Source: CAD feature listing. Evaluate the final solid. Frame: model axes, mm. A direction names the side the tool comes from. Coordinates: 2 decimals unless noted, no trailing zeros. Order: outer loops, then holes, each group sorted by start corner. A loop starts at its lowest first (then second) coordinate and runs counter-clockwise, first axis right, second up.
```python
from build123d import *

# Parameters (mm, degrees)
SKETCH2_R           = 14.5
BOSS_EXTRUDE1_DEPTH = 220
FILLET1_R           = 5
SKETCH3_R           = 19.5
BOSS_EXTRUDE2_DEPTH = 5
FILLET2_R           = 1


with BuildPart() as part:
    # Sketch2 → Boss-Extrude1 (new body)
    with BuildSketch(Plane(origin=(0, 0, 0), x_dir=(1, 0, 0), z_dir=(0, 1, 0))):
        with Locations(Location((0, 0, 0), (0, 0, 270))):
            Circle(SKETCH2_R)
    extrude(amount=BOSS_EXTRUDE1_DEPTH)

    # Fillet1
    fillet1_edges = [part.edges().sort_by_distance(p)[0] for p in [
        (0, 220, -14.5),
    ]]
    fillet(fillet1_edges, radius=FILLET1_R)

    # Sketch3 → Boss-Extrude2 (add)
    with BuildSketch(Plane.XZ):
        with Locations(Location((0, 0, 0), (0, 0, 270))):
            Circle(SKETCH3_R)
    extrude(amount=-BOSS_EXTRUDE2_DEPTH)

    # Fillet2
    fillet2_edges = [part.edges().sort_by_distance(p)[0] for p in [
        (0, 5, 19.5),
        (0, 0, 19.5),
        (0, 5, -14.5),
    ]]
    fillet(fillet2_edges, radius=FILLET2_R)


solid = part.part
```
Q1. Material intervals for line 1 along Y through (x, z) = (-11.5, -13); line 2 along X through (y, z) = (149, -1); line 3 along Y through (x, z) = (11, 8), sorted ascending.
Solutions:
line 1: y = 0 to 5
line 2: x = -14.47 to 14.47
line 3: y = 0 to 217.86
Q2. Section query A-A on x = 0. Output: boundary loops of the cut face in (y, z).
Solutions:
outline: (0, -18.5) arc R1 ccw to (1, -19.5) - (4, -19.5) arc R1 ccw to (5, -18.5) - (5, -15.5) arc R1 cw to (6, -14.5) - (215, -14.5) arc R5 ccw to (220, -9.5) - (220, 9.5) arc R5 ccw to (215, 14.5) - (6, 14.5) arc R1 cw to (5, 15.5) - (5, 18.5) arc R1 ccw to (4, 19.5) - (1, 19.5) arc R1 ccw to (0, 18.5) - close
Q3. Pin query (flat end, axial travel): P1, Ø10, axis at x = 15, z = -11, coming from the -Y side; P2, Ø12, axis at x = -4, y = 88, coming from the -Z side; P3, Ø1, axis at x = -9.5, y = 113.5, coming from the -Z side; P4, Ø6, axis at x = -14.5, z = 3.5, coming from the +Y side. Return the tip coordinate at first contact, or that it passes through.
Solutions:
P1: stops at y = 0
P2: stops at z = -14.5
P3: stops at z = -11.37
P4: stops at y = 219.38
Q4. Section query C-C on y = 178. Output: boundary loops of the cut face in (x, z), plus the area to 3 significant figures.
Solutions:
outline: circle Ø29 at (0, 0)
area: 661 mm2
Q5. Set-up query: faces 1 (the cylindrical face through (19.334, 2.479, 2.539)), 2 (the flat face through (-14, 5, -8)). Return all of +Z, -Z, +X, -X, +Y, -Y with unobstructed straight access to the full face (end or side cutting, diameter ignored); none if empty.
Solutions:
face 1: +Y, -Y
face 2: +Y
Q6. Section query B-B on z = 0. Output: boundary loops of the cut face in (x, y).
Solutions:
outline: (-19.5, 1) arc R1 ccw to (-18.5, 0) - (18.5, 0) arc R1 ccw to (19.5, 1) - (19.5, 4) arc R1 ccw to (18.5, 5) - (15.5, 5) arc R1 cw to (14.5, 6) - (14.5, 215) arc R5 ccw to (9.5, 220) - (-9.5, 220) arc R5 ccw to (-14.5, 215) - (-14.5, 6) arc R1 cw to (-15.5, 5) - (-18.5, 5) arc R1 ccw to (-19.5, 4) - close
